Model file for the job. Use its own axes, mm. A direction names the side the tool comes from. Give positions to 0.01 mm unless a question says otherwise; leave off trailing zeros. Loops run counter-clockwise (first coordinate to the right, second up) from the corner with the lowest first, then second, coordinate; pieces in that order, holes last. Notation, with made-up numbers: (52.5, 73.5) - (91.5, 73.5) arc R25 ccw to (91.5, 101.5) - close; hole circle Ø3 at (73.25, -6.5). An arc over 180 degrees is marked (long way). Use a Markdown table: item, result.
from build123d import *

# Parameters (mm, degrees)
SKETCH1_R                           = 65
BOSS_EXTRUDE1_DEPTH                 = 5
CUT_EXTRUDE2_START                  = -25
CUT_EXTRUDE2_DEPTH                  = 25
FILLET2_R                           = 12
SKETCH9_R                           = 12.5
BOSS_EXTRUDE4_DEPTH                 = 30
SKETCH10_R                          = 4.95
CUT_EXTRUDE3_DEPTH                  = 98.249387408
SKETCH11_W                          = 5
SKETCH11_H                          = 5
CUT_EXTRUDE4_DEPTH                  = 98.249387408
F_1_0MM_DOWEL_HOLE3_D               = 2.8
F_1_0MM_DOWEL_HOLE3_DEPTH           = 33.158795133
F_1_0MM_DOWEL_HOLE3_TIP             = 0.841204867
F_1_0MM_DOWEL_HOLE3_ON_FACE_2_D     = 2.8
F_1_0MM_DOWEL_HOLE3_ON_FACE_2_DEPTH = 33.158795133
F_1_0MM_DOWEL_HOLE3_ON_FACE_2_TIP   = 0.841204867
BOSS_EXTRUDE5_DEPTH                 = 4
BOSS_EXTRUDE5_DEPTH_BACK            = 5
SKETCH13_R                          = 33
F_1_0MM_DOWEL_HOLE4_D               = 9.2
F_1_0MM_DOWEL_HOLE4_DEPTH           = 31.236041152
F_1_0MM_DOWEL_HOLE4_TIP             = 2.763958848
FILLET4_R                           = 15
CUT_EXTRUDE5_DEPTH                  = 98.249387408


with BuildPart() as part:
    # Sketch1 → Boss-Extrude1 (new body)
    with BuildSketch(Plane.XY):
        Circle(SKETCH1_R)
    extrude(amount=BOSS_EXTRUDE1_DEPTH)

    # Sketch6 → Cut-Extrude2 (cut)
    with BuildSketch(Plane.XY.offset(5).offset(CUT_EXTRUDE2_START)):
        with BuildLine():
            ThreePointArc((-65, 0), (-56.291651246, -32.5), (-32.5, -56.291651246))
            ThreePointArc((-32.5, -56.291651246), (-34.303351875, -19.805049439), (-65, 0))
        make_face()
        with BuildLine():
            ThreePointArc((56.291651246, -32.5), (19.805049439, -34.303351875), (0, -65))
            ThreePointArc((0, -65), (32.5, -56.291651246), (56.291651246, -32.5))
        make_face()
        with BuildLine():
            ThreePointArc((0, 65), (-32.5, 56.291651246), (-56.291651246, 32.5))
            ThreePointArc((-56.291651246, 32.5), (-19.805049439, 34.303351875), (0, 65))
        make_face()
        with BuildLine():
            ThreePointArc((32.5, 56.291651246), (34.303351875, 19.805049439), (65, 0))
            ThreePointArc((65, 0), (56.291651246, 32.5), (32.5, 56.291651246))
        make_face()
    extrude(amount=CUT_EXTRUDE2_DEPTH, mode=Mode.SUBTRACT)

    # Fillet2
    fillet2_edges = [part.edges().sort_by_distance(p)[0] for p in [
        (-56.291651246, 32.5, 2.5),
        (0, 65, 2.5),
        (32.5, 56.291651246, 2.5),
        (65, 0, 2.5),
        (-32.5, -56.291651246, 2.5),
        (-65, 0, 2.5),
        (56.291651246, -32.5, 2.5),
        (0, -65, 2.5),
    ]]
    fillet(fillet2_edges, radius=FILLET2_R)

    # Sketch9 → Boss-Extrude4 (add)
    with BuildSketch(Plane(origin=(0, 0, 0), x_dir=(-1, 0, 0), z_dir=(0, 0, -1))):
        Circle(SKETCH9_R)
    extrude(amount=BOSS_EXTRUDE4_DEPTH)

    # Sketch10 → Cut-Extrude3 (cut, through all)
    with BuildSketch(Plane(origin=(0, 0, -30), x_dir=(-1, 0, 0), z_dir=(0, 0, -1))):
        Circle(SKETCH10_R)
    extrude(amount=-CUT_EXTRUDE3_DEPTH, mode=Mode.SUBTRACT)

    # Sketch11 → Cut-Extrude4 (cut, through all)
    with BuildSketch(Plane(origin=(0, 0, -30), x_dir=(-1, 0, 0), z_dir=(0, 0, -1))):
        with Locations((0, 4.95)):
            Rectangle(SKETCH11_W, SKETCH11_H)
    extrude(amount=-CUT_EXTRUDE4_DEPTH, mode=Mode.SUBTRACT)

    # Ø1.0mm Dowel Hole3
    with Locations(Plane(origin=(0, -12.5, -18.578187756), x_dir=(-1, 0, 0), z_dir=(0, -1, 0))):
        with Locations((0, 0)):
            Hole(F_1_0MM_DOWEL_HOLE3_D / 2, depth=F_1_0MM_DOWEL_HOLE3_DEPTH)
            with Locations((0, 0, -(F_1_0MM_DOWEL_HOLE3_DEPTH + F_1_0MM_DOWEL_HOLE3_TIP / 2))):  # 118° drill point
                Cone(0, F_1_0MM_DOWEL_HOLE3_D / 2, F_1_0MM_DOWEL_HOLE3_TIP, mode=Mode.SUBTRACT)

    # Ø1.0mm Dowel Hole3 on face 2
    with Locations(Plane(origin=(12.447431605, 1.14518402, -23.093887112), x_dir=(-0.091614954639, 0.995794506957, 0), z_dir=(0.995794506957, 0.091614954639, 0))):
        with Locations((0, 0)):
            Hole(F_1_0MM_DOWEL_HOLE3_ON_FACE_2_D / 2, depth=F_1_0MM_DOWEL_HOLE3_ON_FACE_2_DEPTH)
            with Locations((0, 0, -(F_1_0MM_DOWEL_HOLE3_ON_FACE_2_DEPTH + F_1_0MM_DOWEL_HOLE3_ON_FACE_2_TIP / 2))):  # 118° drill point
                Cone(0, F_1_0MM_DOWEL_HOLE3_ON_FACE_2_D / 2, F_1_0MM_DOWEL_HOLE3_ON_FACE_2_TIP, mode=Mode.SUBTRACT)

    # Sketch13 → Boss-Extrude5 (add, two sides: drawn at the far end of the back side and taken through both)
    with BuildSketch(Plane(origin=(0, 0, 0), x_dir=(-1, 0, 0), z_dir=(0, 0, -1)).offset(-BOSS_EXTRUDE5_DEPTH_BACK)):
        Circle(SKETCH13_R)
    extrude(amount=BOSS_EXTRUDE5_DEPTH + BOSS_EXTRUDE5_DEPTH_BACK)

    # Ø1.0mm Dowel Hole4
    with Locations(Plane(origin=(11.07745513, 41.341625365, 0), x_dir=(-1, 0, 0), z_dir=(0, 0, -1))):
        with Locations((0, 0), (20.784914346, -84.940934124), (52.862924235, -32.078009888), (-32.078009889, -52.862924235)):
            Hole(F_1_0MM_DOWEL_HOLE4_D / 2, depth=F_1_0MM_DOWEL_HOLE4_DEPTH)
            with Locations((0, 0, -(F_1_0MM_DOWEL_HOLE4_DEPTH + F_1_0MM_DOWEL_HOLE4_TIP / 2))):  # 118° drill point
                Cone(0, F_1_0MM_DOWEL_HOLE4_D / 2, F_1_0MM_DOWEL_HOLE4_TIP, mode=Mode.SUBTRACT)

    # Fillet4
    # the kernel refuses this fillet: 15 mm, written as the material it adds along each edge
    with BuildSketch(Plane(origin=(0, 0, -4), x_dir=(-1, 0, 0), z_dir=(0, 1, 0))) as fillet4_piece_1_section:
        with BuildLine():
            CenterArc((12.5 + FILLET4_R, -FILLET4_R), FILLET4_R, 90, 90)
            Line((12.5, -FILLET4_R), (12.5, 0))
            Line((12.5, 0), (12.5 + FILLET4_R, 0))
        make_face()
    fillet4_piece_1 = revolve(axis=Axis((0, 0, -4), (0, 0, 1)), mode=Mode.PRIVATE)
    fillet4_piece_1 = fillet4_piece_1 - Plane(origin=(0, 0, -18.578187756), x_dir=(1, 0, 0), z_dir=(0, 1, 0)) * Cylinder(1.4, 110, mode=Mode.PRIVATE)
    add(fillet4_piece_1)

    # Sketch17 → Cut-Extrude5 (cut, through all)
    with BuildSketch(Plane(origin=(0, 0, -30), x_dir=(-1, 0, 0), z_dir=(0, 0, -1))):
        with BuildLine():
            Line((2.5, 4.272294466), (2.5, 7.45))
            Line((2.5, 7.45), (-2.5, 7.45))
            Line((-2.5, 7.45), (-2.5, 4.272294466))
            ThreePointArc((-2.5, 4.272294466), (0, -4.95), (2.5, 4.272294466))
        make_face()
    extrude(amount=-CUT_EXTRUDE5_DEPTH, mode=Mode.SUBTRACT)


solid = part.part
(1) Slice it at A-A, the plane z = -27. Write the cut outline in (x, y).
Computed:
| item | result |
|---|---|
| outline | circle Ø25 at (0, 0); hole (-2.5, 4.27) arc R4.95 ccw (long way) to (2.5, 4.27) - (2.5, 7.45) - (-2.5, 7.45) - close |
(2) 3-axis set-ups, long thin cutter, end or side, ignore diameter. For faces 1 (the cylindrical face through (-20.155, 34.104, 2.465)), 2 (the cylindrical face through (-11.923, 3.755, -24.423)), 3 (the flat face through (-2.5, 6, -13)): which of +Z, -Z, +X, -X, +Y, -Y reach the whole face in a straight line?
Computed:
| item | result |
|---|---|
| face 1 | +Z, -Z, +Y |
| face 2 | -Z |
| face 3 | +Z, -Z |
(3) Drill centre lines: probe 1 along Z at (x, y) = (0, -9); probe 2 along Y at (x, z) = (-3, -6); probe 3 along Z at (x, y) = (-23, -52.5). Where is each one in solid material? Low to high. Write a range as [from, to].
Computed:
| item | result |
|---|---|
| probe 1 | [-30, -19.98], [-17.18, 5] |
| probe 2 | [-19.79, -3.94], [3.94, 19.79] |
| probe 3 | [0, 5] |
(4) Slice it at B-B, the plane z = -9.5. Write the cut outline in (x, y).
Computed:
| item | result |
|---|---|
| outline | circle Ø31.78 at (0, 0); hole (-2.5, 4.27) arc R4.95 ccw (long way) to (2.5, 4.27) - (2.5, 7.45) - (-2.5, 7.45) - close |
(5) Pin check, flat tips, straight feed: P1, Ø3, axis at x = 0, z = -18.58, coming from the +Y side; P2, Ø1.5, axis at x = 17.5, y = -4.5, coming from the -Z side; P3, Ø5.5, axis at x = -0.5, z = -4, coming from the -Y side. Stop position of each tip, or through.
Computed:
| item | result |
|---|---|
| P1 | y = 12.62 |
| P2 | z = -7.98 |
| P3 | y = -33 |
(6) Mould opens along Y. For faces 4 (the cylindrical face through (16.896, 62.766, 2.465)), 5 (the flat face through (12, 25, -4)), 6 (the cylindrical face through (8.594, 0.142, -24.336)) say: pulls with the +Y half, pulls with the -Y half, needs draft (parallel to the pull), parting line crosses it, or undercut.
Computed:
| item | result |
|---|---|
| face 4 | pulls with the +Y half |
| face 5 | needs draft |
| face 6 | undercut |
